from build123d import *

# Parameters (mm, degrees)
PLATEOUTLINE_W      = 78.74
PLATEOUTLINE_H      = 78.74
BOSS_EXTRUDE1_DEPTH = 6.35
RAILGUIDES_R        = 4.7625
CUT_EXTRUDE1_DEPTH  = 10
CUT_EXTRUDE2_START  = 5
FUELGRAINMOUNTING_R = 30.1625
CUT_EXTRUDE2_DEPTH  = 5
GASINTAKE_R         = 23.876
CUT_EXTRUDE3_DEPTH  = 5
CUT_EXTRUDE4_START  = 5
SKETCH1_R           = 30.1625
SKETCH1_R_2         = 28.575
CUT_EXTRUDE4_DEPTH  = 1.143


with BuildPart() as part:
    # plateOutline → Boss-Extrude1 (new body)
    with BuildSketch(Plane(origin=(0, 0, 0), x_dir=(1, 0, 0), z_dir=(0, 1, 0))):
        Rectangle(PLATEOUTLINE_W, PLATEOUTLINE_H)
    extrude(amount=BOSS_EXTRUDE1_DEPTH)

    # railGuides → Cut-Extrude1 (cut)
    with BuildSketch(Plane(origin=(0, 0, 0), x_dir=(1, 0, 0), z_dir=(0, 1, 0))):
        with Locations((-30.48, 30.48)):
            Circle(RAILGUIDES_R)
        with Locations((30.48, 30.48)):
            Circle(RAILGUIDES_R)
        with Locations((30.48, -30.48)):
            Circle(RAILGUIDES_R)
        with Locations((-30.48, -30.48)):
            Circle(RAILGUIDES_R)
    extrude(amount=CUT_EXTRUDE1_DEPTH, mode=Mode.SUBTRACT)

    # FuelGrainMounting → Cut-Extrude2 (cut)
    with BuildSketch(Plane(origin=(0, 0, 0), x_dir=(1, 0, 0), z_dir=(0, 1, 0)).offset(CUT_EXTRUDE2_START)):
        Circle(FUELGRAINMOUNTING_R)
    extrude(amount=CUT_EXTRUDE2_DEPTH, mode=Mode.SUBTRACT)

    # GasIntake → Cut-Extrude3 (cut)
    with BuildSketch(Plane(origin=(0, 0, 0), x_dir=(1, 0, 0), z_dir=(0, 1, 0))):
        Circle(GASINTAKE_R)
    extrude(amount=CUT_EXTRUDE3_DEPTH, mode=Mode.SUBTRACT)

    # Sketch1 → Cut-Extrude4 (cut)
    with BuildSketch(Plane(origin=(0, 0, 0), x_dir=(1, 0, 0), z_dir=(0, 1, 0)).offset(CUT_EXTRUDE4_START)):
        Circle(SKETCH1_R)
        Circle(SKETCH1_R_2, mode=Mode.SUBTRACT)
    extrude(amount=-CUT_EXTRUDE4_DEPTH, mode=Mode.SUBTRACT)


solid = part.part
Read the model definition and answer for the solid it produces. Units are mm, in the model's axes. A direction names the side the tool comes from. Round coordinates to 2 decimals unless told otherwise and drop trailing zeros. Order: outer loops, then holes, each group sorted by start corner. A loop starts at its lowest first (then second) coordinate and runs counter-clockwise, first axis right, second up.
1) The part is cut by section C-C on x = 32. Write down the section's boundary in (y, z).
2) Flat-ended cylindrical pins translate along their axes: pin 1 (1.5 mm diameter, centred on x = -14, z = 17, fed in from -Y); pin 2 (12 mm diameter, centred on x = 0, z = -21, fed in from -Y). Find the tip coordinate at first contact, or state that the pin passes through.
3) The mould has two halves that part along Z. Classify faces 1 (the face through (27, 3.857, 11)), 2 (the face through (33.04, 3.131, -34.496)), 3 (the face through (39.37, 3, 1)), 4 (the face through (-1, 3, 39.37)): released by +Z, released by -Z, zero draft, split by the parting line, or undercut.
4) For faces 5 (the face through (-28.547, 4.437, -1.256)), 6 (the face through (-39.37, 3, 1)), determine the directions among +Z, -Z, +X, -X, +Y, -Y from which every point of the face is accessible in a straight line to the end or side of a thin tool.
5) Straight lines are drawn through the part: L1, parallel to X at y = 4.75, z = 30.48; L2, parallel to X at y = 5.2, z = 0. For each, find the intervals that lie inside material, in ascending order.
Resolved:
1. outline: (0, -39.37) - (6.35, -39.37) - (6.35, -34.99) - (0, -34.99) - close; (0, -25.97) - (6.35, -25.97) - (6.35, 25.97) - (0, 25.97) - close; (0, 34.99) - (6.35, 34.99) - (6.35, 39.37) - (0, 39.37) - close
2. pin 1: passes through
2. pin 2: stops at y = 0
3. face 1: undercut
3. face 2: undercut
3. face 3: zero draft
3. face 4: released by +Z
4. face 5: +Y
4. face 6: +Z, -Z, -X, +Y, -Y
5. L1: x = -39.37 to -35.24, -25.72 to 25.72, 35.24 to 39.37
5. L2: x = -39.37 to -30.16, 30.16 to 39.37
